CAD build for the part. Positions are in the model's coordinates, mm. Face numbers are marked on the shaded views. A direction names the side the tool comes from. Round coordinates to 2 decimals unless told otherwise and drop trailing zeros. Order: outer loops, then holes, each group sorted by start corner. A loop starts at its lowest first (then second) coordinate and runs counter-clockwise, first axis right, second up. Notation, with made-up numbers: (55.25, 7.5) - (92.25, 7.5) arc R31 ccw to (92.25, 35.5) - close; hole circle Ø1 at (-2, 59). An arc over 180 degrees is marked (long way). Write item = value, one per line.
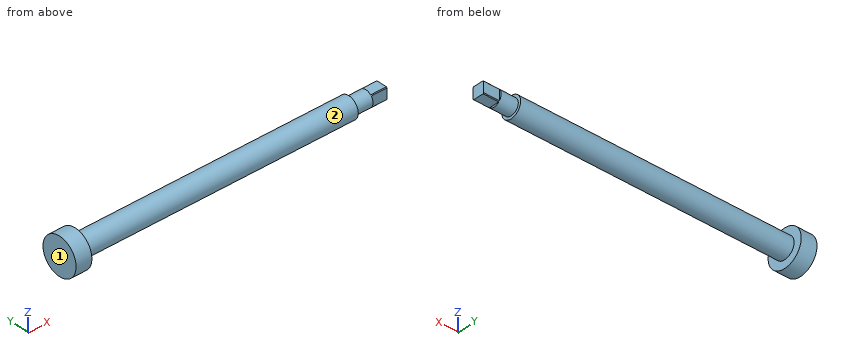
from build123d import *

# Parameters (mm, degrees)
SKETCH2_R          = 9
SKETCH2_W          = 9
SKETCH2_H          = 9
CUT_EXTRUDE1_DEPTH = 12


with BuildPart() as part:
    # Sketch1 → Revolve1 (revolve)
    with BuildSketch(Plane.XY, mode=Mode.PRIVATE) as revolve1_sk:
        Polygon((-12, 0), (-12, 14), (0, 14), (0, 8), (208, 8), (208, 6), (233, 6), (233, 0), align=None)
    revolve(revolve1_sk.sketch.rotate(Axis((500, 0, 0), (-1, 0, 0)), 270), axis=Axis((500, 0, 0), (-1, 0, 0)))

    # Sketch2 → Cut-Extrude1 (cut)
    with BuildSketch(Plane(origin=(221, 0, 0), x_dir=(0, 0, -1), z_dir=(1, 0, 0))):
        Circle(SKETCH2_R)
        Rectangle(SKETCH2_W, SKETCH2_H, mode=Mode.SUBTRACT)
    extrude(amount=CUT_EXTRUDE1_DEPTH, mode=Mode.SUBTRACT)


solid = part.part
(1) Drop flat-ended pins along their axis: pin 1 (6 mm diameter, centred on x = 89, z = -6.5, fed in from -Y); pin 2 (1.2 mm diameter, centred on y = 1, z = 5.5, fed in from +X); pin 3 (4 mm diameter, centred on x = 229.5, z = -0.5, fed in from +Y); pin 4 (1.5 mm diameter, centred on x = 77.5, y = 9.5, fed in from -Z). Give the stop position or say it passes through.
Solved:
pin_1 = -7.19
pin_2 = 221
pin_3 = 4.5
pin_4 = through
(2) Tool access for the marked faces 1 and 2: list every direction of +Z, -Z, +X, -X, +Y, -Y with a clear straight run to the whole face (end or side of a thin tool).
Solved:
face_1 = +Z, -Z, -X, +Y, -Y
face_2 = +X
(3) Band-saw the part on A-A on y = 0. List the corners of the cut face in (x, z).
Solved:
outline = (-12, -14) - (0, -14) - (0, -8) - (208, -8) - (208, -6) - (221, -6) - (221, -4.5) - (233, -4.5) - (233, 4.5) - (221, 4.5) - (221, 6) - (208, 6) - (208, 8) - (0, 8) - (0, 14) - (-12, 14) - close
(4) Band-saw the part on C-C on x = 45. List the corners of the cut face in (y, z), plus the area to 3 significant figures.
Solved:
outline = circle Ø16 at (0, 0)
area = 201 mm²
(5) Band-saw the part on D-D on z = -10. List the corners of the cut face in (x, y).
Solved:
outline = (-12, -9.8) - (0, -9.8) - (0, 9.8) - (-12, 9.8) - close
(6) Probe line 1 along X through (y, z) = (-7.5, 4); line 2 along Y through (x, z) = (99.5, -5.25); line 3 along X through (y, z) = (-5.5, -3.5). List the from-to ranges inside material, lowest first.
Solved:
line_1 = -12 to 0
line_2 = -6.04 to 6.04
line_3 = -12 to 208
